from build123d import *

# Parameters (mm, degrees)
F0_R      = 76.2
F0_R_2    = 50.8
F1_DEPTH  = 69.85
F2_R      = 50.8
F3_DEPTH  = 25.4
F5_R      = 50.8
F6_DEPTH  = 203.2
F7_R      = 76.2
F8_DEPTH  = 25.4
F10_DEPTH = 69.85
F9_R      = 38.1
F11_DEPTH = 203.2


with BuildPart() as f1:
    # F0 (on Top) → F1 (new body, symmetric)
    with BuildSketch(Plane.XY):
        Circle(F0_R)
        Circle(F0_R_2, mode=Mode.SUBTRACT)
    extrude(amount=F1_DEPTH, both=True)

    # F2 (on face) → F3 (join)
    with BuildSketch(Plane.XY.offset(69.85)):
        with BuildLine():
            Line((101.6, 127), (0, 127))
            Line((0, 127), (-101.6, 127))
            ThreePointArc((-101.6, 127), (-119.5605122421, 119.5605122421), (-127, 101.6))
            Line((-127, 101.6), (-127, 0))
            Line((-127, 0), (-127, -101.6))
            ThreePointArc((-127, -101.6), (-119.5605122421, -119.5605122421), (-101.6, -127))
            Line((-101.6, -127), (0, -127))
            Line((0, -127), (101.6, -127))
            ThreePointArc((101.6, -127), (119.5605122421, -119.5605122421), (127, -101.6))
            Line((127, -101.6), (127, 0))
            Line((127, 0), (127, 101.6))
            ThreePointArc((127, 101.6), (119.5605122421, 119.5605122421), (101.6, 127))
        make_face()
        Circle(F2_R, mode=Mode.SUBTRACT)
    extrude(amount=F3_DEPTH)

    # F4: F1 across plane


with BuildPart() as f1_1:
    add(f1.part)
    add(f1.part.mirror(Plane.XY))

    # F5 (on Front) → F6 (join)
    with BuildSketch(Plane.XZ):
        Circle(F5_R)
    extrude(amount=F6_DEPTH)

    # F7 (on face) → F8 (join)
    with BuildSketch(Plane.XZ.offset(203.2)):
        Circle(F7_R)
    extrude(amount=F8_DEPTH)

    # F0 (on Top) → F10 (cut, symmetric)
    with BuildSketch(Plane.XY):
        Circle(F0_R_2)
    extrude(amount=F10_DEPTH, both=True, mode=Mode.SUBTRACT)

    # F9 (on face) → F11 (cut)
    with BuildSketch(Plane.XZ.offset(228.6)):
        Circle(F9_R)
    extrude(amount=-F11_DEPTH, mode=Mode.SUBTRACT)


solid = f1_1.part
Here's how the part is built. I have some questions about the finished solid (model axes, mm). A direction names the side the tool comes from. Round coordinates to 2 decimals unless told otherwise and drop trailing zeros. Order: outer loops, then holes, each group sorted by start corner. A loop starts at its lowest first (then second) coordinate and runs counter-clockwise, first axis right, second up. Notation, with made-up numbers: M 85,-0.5 L 134,-0.5 A12 cw 134,10.5 Z; hole C -1,13 d10. An arc over 180 degrees is marked long. Return JSON: item names as keys, results as strings. Group by question number.
1. If we section it at C-C on z = 59: List the corners of the cut face in (x, y) for me.
2. If we mould it in two halves opening along Y, with no side actions, what happens to faces 4 (the face through (48.454, -128.973, 15.259)), 5 (the face through (55, 2, 95.25)), 6 (the face through (119.36, -119.76, 82.37)), 7 (the face through (-119.36, 119.76, -82.37))? For each: pulls with the +Y half, pulls with the -Y half, needs draft (parallel to the pull), parting line crosses it, or undercut.
3. If we section it at B-B on y = 0: List the corners of the cut face in (x, z) for me.
4. If we section it at D-D on y = -118.5: List the corners of the cut face in (x, z) for me, then the cut area to 3 significant figures.
5. On a 3-axis mill with a long thin cutter (end or side, diameter ignored), from which of +Z, -Z, +X, -X, +Y, -Y can I reach the whole of each face in a straight line? I mean faces 1 (the face through (55, -55, 69.85)), 2 (the face through (-38.063, -132.466, 1.675)), 3 (the face through (-127, 1, -82)). Say none if no direction works.
6. I'm going to push flat-ended pins straight in: pin 1 Ø6 at (x, z) = (-76, 12.5) entering from -Y; pin 2 Ø12.5 at (x, z) = (-38.5, 88.5) entering from -Y; pin 3 Ø1.5 at (x, y) = (37.5, -192) entering from +Z; pin 4 Ø5 at (x, y) = (-3, -140) entering from -Z. Where does each tip first touch, or does it pass through?
7. If we section it at A-A on x = 0: List the corners of the cut face in (y, z) for me, then the cut area to 3 significant figures.
8. Please list where these lines run through material, in increasing order: probe 1 along Z at (x, y) = (0, -105.5); probe 2 along Z at (x, y) = (-18, 105); probe 3 along Z at (x, y) = (0, -130.5).
Reply:
{
 "1": {"outline": "C 0,0 d152.4; M -48.22,-228.6 L 48.22,-228.6 L 48.22,-203.2 L -48.22,-203.2 Z; hole C 0,0 d101.6"},
 "2": {"face 4": "undercut", "face 5": "needs draft", "face 6": "pulls with the -Y half", "face 7": "pulls with the +Y half"},
 "3": {"outline": "M -127,-95.25 L -50.8,-95.25 L -50.8,95.25 L -127,95.25 L -127,69.85 L -76.2,69.85 L -76.2,-69.85 L -127,-69.85 Z; M 50.8,-95.25 L 127,-95.25 L 127,-69.85 L 76.2,-69.85 L 76.2,69.85 L 127,69.85 L 127,95.25 L 50.8,95.25 Z"},
 "4": {"outline": "M -120.56,-95.25 L 120.56,-95.25 L 120.56,-69.85 L -120.56,-69.85 Z; M -120.56,69.85 L 120.56,69.85 L 120.56,95.25 L -120.56,95.25 Z; C 0,0 d101.6; hole C 0,0 d76.2", "area": "15,800 mm^2"},
 "5": {"face 1": "none", "face 2": "-Y", "face 3": "+Z, -Z, -X, +Y, -Y"},
 "6": {"pin 1": "y = -228.6", "pin 2": "y = -127", "pin 3": "z = 35.07", "pin 4": "z = -50.8"},
 "7": {"outline": "M -228.6,-76.2 L -203.2,-76.2 L -203.2,-50.8 L -76.2,-50.8 L -76.2,-69.85 L -127,-69.85 L -127,-95.25 L -50.8,-95.25 L -50.8,-38.1 L -228.6,-38.1 Z; M -228.6,38.1 L -50.8,38.1 L -50.8,95.25 L -127,95.25 L -127,69.85 L -76.2,69.85 L -76.2,50.8 L -203.2,50.8 L -203.2,76.2 L -228.6,76.2 Z; M 50.8,-95.25 L 127,-95.25 L 127,-69.85 L 76.2,-69.85 L 76.2,69.85 L 127,69.85 L 127,95.25 L 50.8,95.25 Z", "area": "18,100 mm^2"},
 "8": {"probe 1": "-95.25 to -69.85, -50.8 to -38.1, 38.1 to 50.8, 69.85 to 95.25", "probe 2": "-95.25 to -69.85, 69.85 to 95.25", "probe 3": "-50.8 to -38.1, 38.1 to 50.8"}
}
